Can you work these out from the model? Positions are in its coordinate system, mm. Face numbers are marked on the shaded views. Round coordinates to 2 decimals unless told otherwise and drop trailing zeros. Loops run counter-clockwise (first coordinate to the right, second up) from the corner with the lowest first, then second, coordinate; pieces in that order, holes last. Notation, with made-up numbers: M 50,-35 L 78,-35 A15 ccw 78,-12 Z; hole C 4.25,49.25 d7. An arc over 180 degrees is marked long. Return JSON: item names as keys, results as strings.
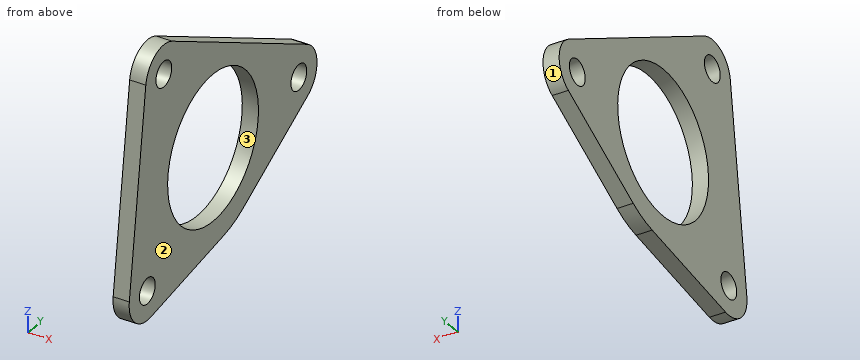
Autodesk Inventor part; units mm, degrees
ref_plane "YZ Plane" through (0, 0, 0) normal (1, 0, 0) x (0, 1, 0)
ref_plane "XZ Plane" through (0, 0, 0) normal (0, 1, 0) x (-1, 0, 0)
ref_plane "XY Plane" through (0, 0, 0) normal (0, 0, 1) x (1, 0, 0)
sketch "Sketch1" plane through (0, 0, 0) normal (1, 0, 0) x (0, 1, 0)
  line L0 (-15.4794, 22.1069) -> (0, 0) construction
  line L1 (0, 0) -> (26.9875, 0) construction
  line L2 (0, 0) -> (-20.6736, -17.3472) construction
  arc A0 (-12.8405, 27.1761) -> (-21.1455, 22.8528) centre (-15.4794, 22.1069) ccw
  arc A1 (-26.3397, -16.6013) -> (-19.6431, -22.9686) centre (-20.6736, -17.3472) ccw
  arc A2 (29.8114, -4.9686) -> (29.6264, 5.0693) centre (26.9875, 0) ccw
  circle A3 centre (0, 0) radius 14.2875 construction
  line L3 (9.4129, -16.562) -> (29.8114, -4.9686)
  arc A4 (3.4351, -18.7377) -> (9.4129, -16.562) centre (0, 0) ccw
  line L4 (3.4351, -18.7377) -> (-19.6431, -22.9686)
  line L5 (-26.3397, -16.6013) -> (-21.1455, 22.8528)
  line L6 (-12.8405, 27.1761) -> (29.6264, 5.0693)
  line L7 (0, 0) -> (0, -5.4993)
  dimension "d0" = 26.9875
  dimension "d1" = 95
  dimension "d2" = 5.715
  dimension "d3" = 28.575
  dimension "d22" = 19.05
  dimension "d23" = 50
extrude "Plate1" add sketch "Sketch1" along normal blind 3.175
hole "Hole1" at (0, 0, 0) direction (1, 0, 0) diameter 28.575 depth 3.175 tip angle 118
hole "Hole2" at (0, 26.9875, 0) at (0, -15.4794, 22.1069) at (0, -20.6736, -17.3472) direction (1, 0, 0) diameter 4.9784 depth 3.175 tip angle 118
equation "\"d11\" = Thickness"
equation "\"d18\" = Thickness"
equation "\"d5\" = Thickness"
equation "\"BendRadius\" = Thickness"
equation "\"BendReliefWidth\" = Thickness"
equation "\"BendReliefDepth\" = 0.5 * Thickness"
equation "\"CornerReliefSize\" = 4 * Thickness"
equation "\"MinimumRemnant\" = 2 * Thickness"
equation "\"TransitionRadius\" = BendRadius"
equation "\"JacobiRadiusSize\" = BendRadius"
equation "\"GapSize\" = Thickness"
properties part number "PLATE,REVERSER,SUPPORT" material "Aluminum 6061"
Q1. Suppose I cut it at A-A, the plane y = 0. Please give me the cut outline in (x, z) (1 decimal), plus the area to 3 significant figures.
Results:
{"outline": "M 0,-19.4 L 3.2,-19.4 L 3.2,-14.3 L 0,-14.3 Z; M 0,14.3 L 3.2,14.3 L 3.2,20.5 L 0,20.5 Z", "area": "35.8 mm2"}
Q2. If I drill on line 1 along Y through (x, z) = (0.75, -4); line 2 along Z through (x, y) = (0.2, -1); line 3 along Z through (x, y) = (1.8, -11), over which ranges is the centre line in solid material (lowest first)?
Results:
{"line 1": "y = -24.68 to -13.72, 13.72 to 31.07", "line 2": "z = -19.55 to -14.25, 14.25 to 21.01", "line 3": "z = -21.38 to -9.12, 9.12 to 26.22"}
Q3. Suppose I cut it at B-B, the plane x = 1.85. Please give me the cut outline in (y, z) (1 decimal), plus the area to 3 significant figures.
Results:
{"outline": "M -26.3,-16.6 A5.7 ccw -19.6,-23 L 3.4,-18.7 A19.1 ccw 9.4,-16.6 L 29.8,-5 A5.7 ccw 29.6,5.1 L -12.8,27.2 A5.7 ccw -21.1,22.9 Z; hole C -20.7,-17.3 d5; hole C -15.5,22.1 d5; hole C 0,0 d28.6; hole C 27,0 d5", "area": "1,200 mm2"}
Q4. I'm going to push a flat-ended pin straight in: pin 1 Ø3 at (y, z) = (-20.67, -17.35) entering from -X. Where does the tip first touch, or does it pass through?
Results:
{"pin 1": "passes through"}
Q5. Suppose I cut it at C-C, the plane z = 10.5. Please give me the cut outline in (x, y) (3 decimals).
Results:
{"outline": "M 0,-22.772 L 3.175,-22.772 L 3.175,-9.689 L 0,-9.689 Z; M 0,9.689 L 3.175,9.689 L 3.175,19.194 L 0,19.194 Z"}
Q6. Suppose I cut it at D-D, the plane z = 0. Please give me the cut outline in (x, y) (1 decimal).
Results:
{"outline": "M 0,-24.2 L 3.2,-24.2 L 3.2,-14.3 L 0,-14.3 Z; M 0,14.3 L 3.2,14.3 L 3.2,24.5 L 0,24.5 Z; M 0,29.5 L 3.2,29.5 L 3.2,32.7 L 0,32.7 Z"}
Q7. Thinking about a two-plate mould opening in Z: for the marked faces 1, 2 and 3, which applies, pulls with the +Z half, pulls with the -Z half, needs draft (parallel to the pull), parting line crosses it, or undercut?
Results:
{"face 1": "parting line crosses it", "face 2": "needs draft", "face 3": "undercut"}
